Can you work these out from the model? Positions are in its coordinate system, mm. Give positions to 0.01 mm unless a question says otherwise; leave off trailing zeros. Order: outer loops, then holes, each group sorted by start corner. A loop starts at its lowest first (then second) coordinate and runs counter-clockwise, first axis right, second up. Notation, with made-up numbers: (1.25, -12.5) -> (30.25, -12.5) arc R21 ccw to (30.25, 24.5) -> close; hole circle Ø5 at (-2, -5). An arc over 180 degrees is marked (long way). Answer as CSV lines item,"result".
```python
from build123d import *

# Parameters (mm, degrees)
BOSS_EXTRUDE1_DEPTH = 80


with BuildPart() as part:
    # Sketch1 → Boss-Extrude1 (new body)
    with BuildSketch(Plane.XY):
        with BuildLine():
            Line((6, 0), (6.4, 1.85))
            Line((6.4, 1.85), (6, 1.85))
            Line((6, 1.85), (6, 2.35))
            Line((6, 2.35), (7.15, 3.45))
            Line((7.15, 3.45), (6, 3.45))
            Line((6, 3.45), (0, 3.45))
            Line((0, 3.45), (-1.15, 3.45))
            Line((-1.15, 3.45), (0, 2.35))
            Line((0, 2.35), (0, 1.85))
            Line((0, 1.85), (-0.4, 1.85))
            Line((-0.4, 1.85), (0, 0))
            Line((0, 0), (1, 0))
            Line((1, 0), (1, 1.6))
            ThreePointArc((1, 1.6), (1.146446609, 1.953553391), (1.5, 2.1))
            Line((1.5, 2.1), (4.5, 2.1))
            ThreePointArc((4.5, 2.1), (4.853553391, 1.953553391), (5, 1.6))
            Line((5, 1.6), (5, 0))
            Line((5, 0), (6, 0))
        make_face()
    extrude(amount=BOSS_EXTRUDE1_DEPTH)


solid = part.part
```
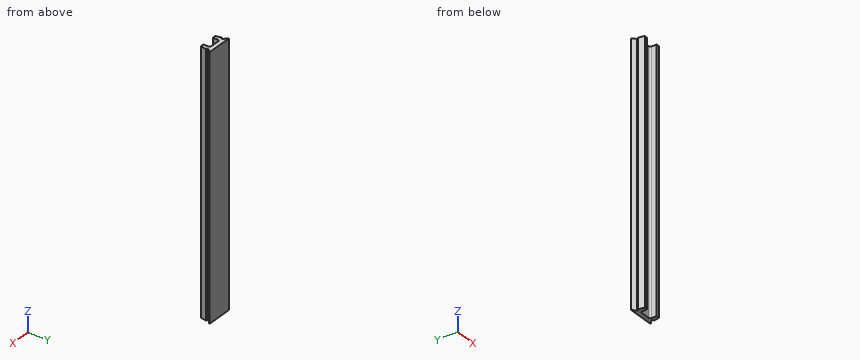
Item 1: For pin 1 (1 mm diameter, centred on x = -0.5, y = 1, fed in from +Z); pin 2 (2.5 mm diameter, centred on x = 3, z = 42.5, fed in from -Y); pin 3 (1 mm diameter, centred on y = 0.5, z = 58, fed in from -X); pin 4 (1 mm diameter, centred on y = 1.5, z = 14, fed in from +X), each with a flat end and sliding along its axis, tell me the tip position at first contact or that it passes through.
Numbers:
pin 1,"stops at z = 80"
pin 2,"stops at y = 2.1"
pin 3,"stops at x = -0.22"
pin 4,"stops at x = 6.4"
Item 2: Imagine slicing it at A-A, the plane y = 0.9. Please give me the cut outline in (x, z).
Numbers:
outline,"(-0.19, 0) -> (1, 0) -> (1, 80) -> (-0.19, 80) -> close; (5, 0) -> (6.19, 0) -> (6.19, 80) -> (5, 80) -> close"
Item 3: Please list where these lines run through material, in increasing order: line 1 along X through (y, z) = (2.35, 35.5); line 2 along Y through (x, z) = (3.5, 28); line 3 along X through (y, z) = (1.8, 33.5).
Numbers:
line 1,"x = 0 to 6"
line 2,"y = 2.1 to 3.45"
line 3,"x = -0.39 to 1.04, 4.96 to 6.39"
Item 4: Imagine slicing it at C-C, the plane x = 3. Please give me the cut outline in (y, z).
Numbers:
outline,"(2.1, 0) -> (3.45, 0) -> (3.45, 80) -> (2.1, 80) -> close"
Item 5: Imagine slicing it at B-B, the plane z = 31.5. Please give me the cut outline in (x, y).
Numbers:
outline,"(-1.15, 3.45) -> (0, 2.35) -> (0, 1.85) -> (-0.4, 1.85) -> (0, 0) -> (1, 0) -> (1, 1.6) arc R0.5 cw to (1.5, 2.1) -> (4.5, 2.1) arc R0.5 cw to (5, 1.6) -> (5, 0) -> (6, 0) -> (6.4, 1.85) -> (6, 1.85) -> (6, 2.35) -> (7.15, 3.45) -> close"
